Drawing for the job (mm, zero at the part's lowest x, y, z). Coordinates: 2 decimals unless noted, no trailing zeros. Loops run counter-clockwise (first coordinate to the right, second up) from the corner with the lowest first, then second, coordinate; pieces in that order, holes last. Notation, with made-up numbers: (51.5, 20) -> (109.5, 20) arc R6 ccw to (109.5, 29) -> close; hole circle Ø2 at (-10, 66.25). An arc over 180 degrees is marked (long way). Write each question's results on one line, items separated by ' | '.
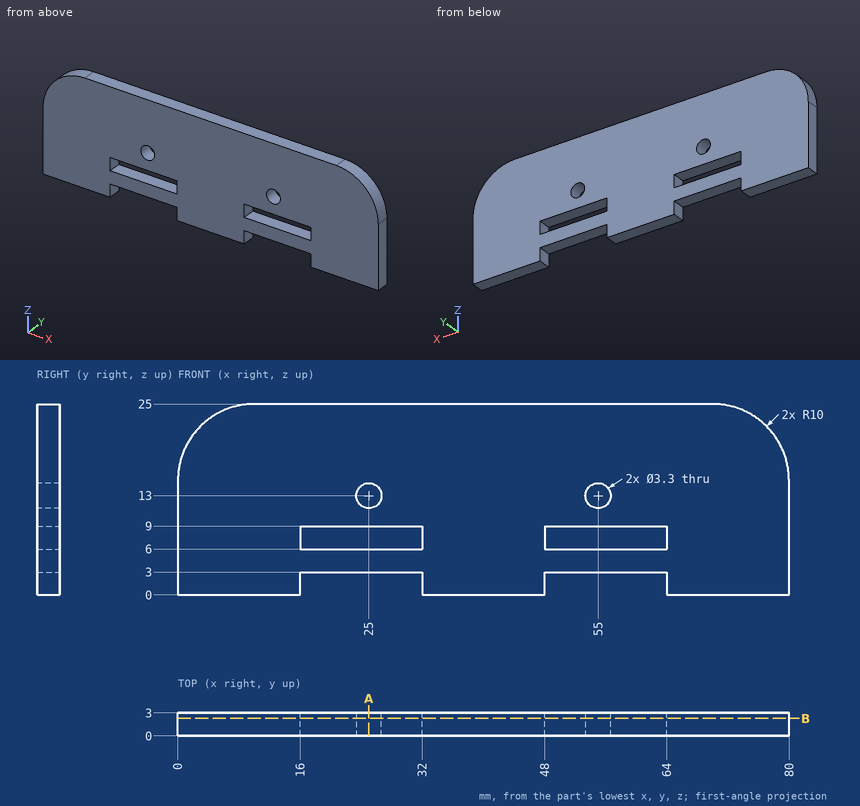
1) Drill centre lines: L1, parallel to X at y = 2.2, z = 13; L2, parallel to Z at x = 25, y = 0.6; L3, parallel to X at y = 2.9, z = 6.75. Where is each one in solid material? Low to high. Write a range as from..to.
Outcome:
L1: x = 0..23.35, 26.65..53.35, 56.65..80 | L2: z = 3..6, 9..11.35, 14.65..25 | L3: x = 0..16, 32..48, 64..80
2) Slice it at B-B (y = 2.3). Write the cut outline in (x, z), then the cut area to 3 significant figures.
Outcome:
outline: (0, 0) -> (16, 0) -> (16, 3) -> (32, 3) -> (32, 0) -> (48, 0) -> (48, 3) -> (64, 3) -> (64, 0) -> (80, 0) -> (80, 15) arc R10 ccw to (70, 25) -> (10, 25) arc R10 ccw to (0, 15) -> close; hole (16, 6) -> (32, 6) -> (32, 9) -> (16, 9) -> close; hole circle Ø3.3 at (25, 13); hole (48, 6) -> (64, 6) -> (64, 9) -> (48, 9) -> close; hole circle Ø3.3 at (55, 13) | area: 1,750 mm^2
3) Pin check, flat tips, straight feed: pin 1 (0.9 mm diameter, centred on y = 1.5, z = 1.5, fed in from -X); pin 2 (1.5 mm diameter, centred on x = 54.5, y = 1.5, fed in from -Z); pin 3 (1 mm diameter, centred on y = 2, z = 21, fed in from -X). Stop position of each tip, or through.
Outcome:
pin 1: stops at x = 0 | pin 2: stops at z = 3 | pin 3: stops at x = 1.65
4) Slice it at A-A (x = 25). Write the cut outline in (y, z).
Outcome:
outline: (0, 3) -> (3, 3) -> (3, 6) -> (0, 6) -> close; (0, 9) -> (3, 9) -> (3, 11.35) -> (0, 11.35) -> close; (0, 14.65) -> (3, 14.65) -> (3, 25) -> (0, 25) -> close
